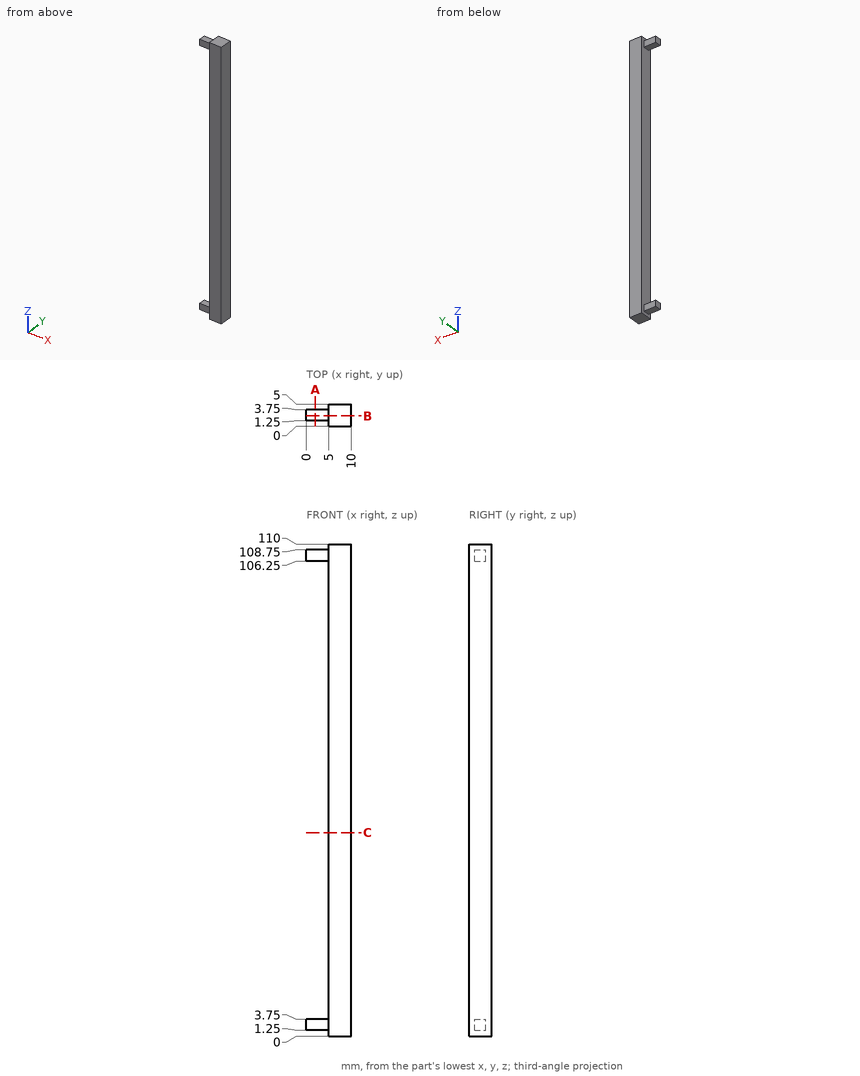
Drawing for the job (mm, zero at the part's lowest x, y, z). Round coordinates to 2 decimals unless told otherwise and drop trailing zeros. Order: outer loops, then holes, each group sorted by start corner. A loop starts at its lowest first (then second) coordinate and runs counter-clockwise, first axis right, second up. Notation, with made-up numbers: (87.5, -23.5) -> (130.5, -23.5) arc R21 ccw to (130.5, -10.5) -> close; hole circle Ø1 at (14.25, -7). An arc over 180 degrees is marked (long way). Write item = value, one per line. Start each with the question number.
(1) Cut at A-A, the plane x = 2. List the corners of the cut face in (y, z), then the cut area to 3 significant figures.
(2) Probe line 1 (X direction, y = 1.95, z = 52); line 2 (Z direction, x = 4, y = 3.65). List the from-to ranges inside material, lowest first. Write a range as [from, to].
(3) Cut at C-C, the plane z = 45.5. List the corners of the cut face in (x, y).
(4) Pin check, flat tips, straight feed: P1, Ø2, axis at x = 1.5, y = 2.5, coming from the -Z side; P2, Ø1.2, axis at x = 2.5, y = 2.5, coming from the +Z side; P3, Ø1, axis at y = 4.5, z = 57, coming from the -X side. Stop position of each tip, or through.
(5) Cut at B-B, the plane y = 2.35. List the corners of the cut face in (x, z).
Model answer:
q1.outline = (1.25, 1.25) -> (3.75, 1.25) -> (3.75, 3.75) -> (1.25, 3.75) -> close; (1.25, 106.25) -> (3.75, 106.25) -> (3.75, 108.75) -> (1.25, 108.75) -> close
q1.area = 12.5 mm2
q2.line_1 = [5, 10]
q2.line_2 = [1.25, 3.75], [106.25, 108.75]
q3.outline = (5, 0) -> (10, 0) -> (10, 5) -> (5, 5) -> close
q4.P1 = 1.25
q4.P2 = 108.75
q4.P3 = 5
q5.outline = (0, 1.25) -> (5, 1.25) -> (5, 0) -> (10, 0) -> (10, 110) -> (5, 110) -> (5, 108.75) -> (0, 108.75) -> (0, 106.25) -> (5, 106.25) -> (5, 3.75) -> (0, 3.75) -> close
